```python
from build123d import *

# Parameters (mm, degrees)
SZKIC1_R                    = 1.35
DODANIE_WYCI_GNI_CIE1_DEPTH = 5
DODANIE_WYCI_GNI_CIE2_DEPTH = 25
SZKIC8_W                    = 8
SZKIC8_H                    = 5
SZKIC8_W_2                  = 9
DODANIE_WYCI_GNI_CIE3_DEPTH = 25
SZKIC1_4_R                  = 1.35
DODANIE_WYCI_GNI_CIE4_DEPTH = 3


with BuildPart() as part:
    # Szkic1 → Dodanie-wyci_gni_cie1 (new body)
    with BuildSketch(Plane(origin=(0, 0, 0), x_dir=(1, 0, 0), z_dir=(0, 1, 0))):
        Polygon((-20.5, 55.3963255), (19.595579106, 55.3963255), (24.347789553, 80.533497461), (24.347789553, 126.117958863), (24.347789553, 131.76713902), (24.347789553, 149.567063292), (15.53266243, 139.1963255), (-16.437083324, 139.1963255), (-25.252210447, 149.567063292), (-25.252210447, 131.76713902), (-25.252210447, 126.117958863), (-25.252210447, 80.533497461), align=None)
        Polygon((-13.152210447, 117.3963255), (-12.652210447, 117.3963255), (11.747789553, 117.3963255), (12.247789553, 117.3963255), (17.347789553, 112.070622628), (17.347789553, 72.740102496), (12.295579106, 66.7963255), (-13.2, 66.7963255), (-18.252210447, 72.740102496), (-18.252210447, 112.070622628), align=None, mode=Mode.SUBTRACT)
        Polygon((15.53266243, 139.1963255), (24.347789553, 149.567063292), (24.347789553, 194.281753518), (15.236444388, 203.7963255), (-16.140865282, 203.7963255), (-25.252210447, 194.281753518), (-25.252210447, 149.567063292), (-16.437083324, 139.1963255), align=None)
        Polygon((-13.152210447, 196.7963255), (-12.652210447, 196.7963255), (11.747789553, 196.7963255), (12.247789553, 196.7963255), (17.347789553, 191.470622628), (17.347789553, 152.140102496), (12.295579106, 146.1963255), (-13.2, 146.1963255), (-18.252210447, 152.140102496), (-18.252210447, 191.470622628), align=None, mode=Mode.SUBTRACT)
        Polygon((-12.652210447, 151.7963255), (-12.652210447, 196.7963255), (-13.152210447, 196.7963255), (-18.252210447, 191.470622628), (-18.252210447, 152.140102496), (-13.2, 146.1963255), (12.295579106, 146.1963255), (17.347789553, 152.140102496), (17.347789553, 191.470622628), (12.247789553, 196.7963255), (11.747789553, 196.7963255), (11.747789553, 151.7963255), align=None)
        with Locations(Location((-15.404420894, 155.2963255, 0), (0, 0, 270))):
            Circle(SZKIC1_R, mode=Mode.SUBTRACT)
        with Locations(Location((-8.952210447, 148.9963255, 0), (0, 0, 270))):
            Circle(SZKIC1_R, mode=Mode.SUBTRACT)
        with Locations(Location((-15.404420894, 172.2963255, 0), (0, 0, 270))):
            Circle(SZKIC1_R, mode=Mode.SUBTRACT)
        with Locations(Location((-15.452210447, 189.2963255, 0), (0, 0, 270))):
            Circle(SZKIC1_R, mode=Mode.SUBTRACT)
        with Locations(Location((8.047789553, 148.9963255, 0), (0, 0, 270))):
            Circle(SZKIC1_R, mode=Mode.SUBTRACT)
        with Locations(Location((14.5, 155.2963255, 0), (0, 0, 270))):
            Circle(SZKIC1_R, mode=Mode.SUBTRACT)
        with Locations(Location((14.5, 172.2963255, 0), (0, 0, 270))):
            Circle(SZKIC1_R, mode=Mode.SUBTRACT)
        with Locations(Location((14.547789553, 189.2963255, 0), (0, 0, 270))):
            Circle(SZKIC1_R, mode=Mode.SUBTRACT)
    extrude(amount=DODANIE_WYCI_GNI_CIE1_DEPTH)

    # Szkic1_3 → Dodanie-wyci_gni_cie2 (add)
    with BuildSketch(Plane(origin=(0, 0, 0), x_dir=(1, 0, 0), z_dir=(0, 1, 0))):
        Polygon((-20.5, 55.3963255), (19.595579106, 55.3963255), (24.347789553, 80.533497461), (24.347789553, 194.281753518), (15.236444388, 203.7963255), (-16.140865282, 203.7963255), (-25.252210447, 194.281753518), (-25.252210447, 80.533497461), align=None)
        Polygon((-13.152210447, 117.3963255), (12.247789553, 117.3963255), (17.347789553, 112.070622628), (17.347789553, 72.740102496), (12.295579106, 66.7963255), (-13.2, 66.7963255), (-18.252210447, 72.740102496), (-18.252210447, 112.070622628), align=None, mode=Mode.SUBTRACT)
        Polygon((12.247789553, 196.7963255), (17.347789553, 191.470622628), (17.347789553, 152.140102496), (12.295579106, 146.1963255), (-13.2, 146.1963255), (-18.252210447, 152.140102496), (-18.252210447, 191.470622628), (-13.152210447, 196.7963255), align=None, mode=Mode.SUBTRACT)
    extrude(amount=DODANIE_WYCI_GNI_CIE2_DEPTH)

    # Szkic8 → Dodanie-wyci_gni_cie3 (add)
    with BuildSketch(Plane(origin=(0, 25, 0), x_dir=(1, 0, 0), z_dir=(0, 1, 0))):
        Polygon((19.595579106, 51.744454691), (19.595579106, 55.3963255), (12.595579106, 55.3963255), (12.595579106, 50.3963255), (16.925579106, 50.3963255), align=None)
        with Locations((0.758846465, 52.8963255)):
            Rectangle(SZKIC8_W, SZKIC8_H)
        with Locations((-16, 52.8963255)):
            Rectangle(SZKIC8_W_2, SZKIC8_H)
    extrude(amount=-DODANIE_WYCI_GNI_CIE3_DEPTH)

    # Szkic1_4 → Dodanie-wyci_gni_cie4 (add)
    with BuildSketch(Plane(origin=(0, 0, 0), x_dir=(1, 0, 0), z_dir=(0, 1, 0))):
        Polygon((-12.652210447, 72.3963255), (-12.652210447, 117.3963255), (-13.152210447, 117.3963255), (-18.252210447, 112.070622628), (-18.252210447, 72.740102496), (-13.2, 66.7963255), (12.295579106, 66.7963255), (17.347789553, 72.740102496), (17.347789553, 112.070622628), (12.247789553, 117.3963255), (11.747789553, 117.3963255), (11.747789553, 72.3963255), align=None)
        with Locations(Location((-15.404420894, 75.8963255, 0), (0, 0, 270))):
            Circle(SZKIC1_4_R, mode=Mode.SUBTRACT)
        with Locations(Location((-8.952210447, 69.5963255, 0), (0, 0, 270))):
            Circle(SZKIC1_4_R, mode=Mode.SUBTRACT)
        with Locations(Location((-15.404420894, 92.8963255, 0), (0, 0, 270))):
            Circle(SZKIC1_4_R, mode=Mode.SUBTRACT)
        with Locations(Location((-15.452210447, 109.8963255, 0), (0, 0, 270))):
            Circle(SZKIC1_4_R, mode=Mode.SUBTRACT)
        with Locations(Location((8.047789553, 69.5963255, 0), (0, 0, 270))):
            Circle(SZKIC1_4_R, mode=Mode.SUBTRACT)
        with Locations(Location((14.5, 75.8963255, 0), (0, 0, 270))):
            Circle(SZKIC1_4_R, mode=Mode.SUBTRACT)
        with Locations(Location((14.5, 92.8963255, 0), (0, 0, 270))):
            Circle(SZKIC1_4_R, mode=Mode.SUBTRACT)
        with Locations(Location((14.547789553, 109.8963255, 0), (0, 0, 270))):
            Circle(SZKIC1_4_R, mode=Mode.SUBTRACT)
    extrude(amount=DODANIE_WYCI_GNI_CIE4_DEPTH)


solid = part.part
```
Could you check a few things on this model? Use its own coordinates, in mm. A direction names the side the tool comes from. Give positions to 0.01 mm unless a question says otherwise; leave off trailing zeros. Loops run counter-clockwise (first coordinate to the right, second up) from the corner with the lowest first, then second, coordinate; pieces in that order, holes last. Notation, with made-up numbers: (5.5, 63) -> (64.5, 63) arc R9 cw to (64.5, 75) -> close; hole circle Ø10 at (3, -17). An arc over 180 degrees is marked (long way). Put each result on its own line as item: value.
(1) For faces 5 (the face through (0, 2, -151.796)), 6 (the face through (19.596, 13, -54)), 7 (the face through (12.596, 13, -53)), 8 (the face through (0, 14, -66.796)), which set-ups out of +Z, -Z, +X, -X, +Y, -Y let a thin tool reach every point of the face, with its end or its side?
Computed:
face 5: +Y, -Y
face 6: +Z, +X, +Y, -Y
face 7: +Z, +Y, -Y
face 8: +Y
(2) I'm going to push flat-ended pins straight in: pin 1 Ø18 at (x, z) = (-7.5, -180.5) entering from +Y; pin 2 Ø1.6 at (x, z) = (-15.45, -189.3) entering from -Y; pin 3 Ø2.5 at (x, y) = (-6, 14) entering from +Z; pin 4 Ø6 at (y, z) = (15, -75.5) entering from -X. Where does each tip first touch, or does it pass through?
Computed:
pin 1: y = 5
pin 2: through
pin 3: z = -55.4
pin 4: x = -24.87
(3) Thinking about a two-plate mould opening in Z: for faces 1 (the face through (14.559, 2.465, -173.645)), 2 (the face through (19.86, 12.32, -198.97)), 3 (the face through (-1, 25, -128)), 4 (the face through (-15, 1.48, -74.61)), which applies, pulls with the +Z half, pulls with the -Z half, needs draft (parallel to the pull), parting line crosses it, or undercut?
Computed:
face 1: undercut
face 2: pulls with the -Z half
face 3: needs draft
face 4: undercut
(4) Imagine slicing it at B-B on y = 10.25. State how many separate pieces and enclosed holes the cut face has, plus the area to 3 significant figures.
Computed:
separate pieces: 1
enclosed holes: 2
area: 3,780 mm^2
(5) Please list where these lines run through material, in increasing order: probe 1 along Z at (x, y) = (-4.5, 1.75); probe 2 along Z at (x, y) = (8.5, 10.25); probe 3 along X at (y, z) = (6.75, -177). Write a range as [from, to].
Computed:
probe 1: [-203.8, -196.8], [-151.8, -117.4], [-72.4, -55.4]
probe 2: [-203.8, -196.8], [-146.2, -117.4], [-66.8, -55.4]
probe 3: [-25.25, -18.25], [17.35, 24.35]
(6) Imagine slicing it at A-A on z = -182. Write out the boundary of the cut face in (x, y), plus the area to 3 significant figures.
Computed:
outline: (-25.25, 0) -> (-12.65, 0) -> (-12.65, 5) -> (-18.25, 5) -> (-18.25, 25) -> (-25.25, 25) -> close; (11.75, 0) -> (24.35, 0) -> (24.35, 25) -> (17.35, 25) -> (17.35, 5) -> (11.75, 5) -> close
area: 406 mm^2
